from build123d import *

# Parameters (mm, degrees)
SKETCH_1_W               = 250
SKETCH_1_H               = 250
EXTRUDE_1_DEPTH          = 3
HOLE_WIZARD_1_D          = 3.3
PATTERN_CIRCULAR_1_COUNT = 6
SKETCH_5_R               = 22.5
CUT_EXTRUDE_1_DEPTH      = 10


with BuildPart() as part:
    # 草图1 → 凸台-拉伸1 (new body)
    with BuildSketch(Plane(origin=(0, 0, 0), x_dir=(1, 0, 0), z_dir=(0, 1, 0))):
        Rectangle(SKETCH_1_W, SKETCH_1_H)
    extrude(amount=EXTRUDE_1_DEPTH)

    # 孔1 (through all)
    with Locations(Plane(origin=(0, 3, 0), x_dir=(1, 0, 0), z_dir=(0, 1, 0))):
        with Locations((0, -48)):
            hole_wizard_1 = Hole(HOLE_WIZARD_1_D / 2)

    # 阵列(圆周)1: 孔1 ×6 about axis
    pattern_circular_1_axis = Axis((0, 0, 76.5), (0, 1, 0))
    for i in range(1, PATTERN_CIRCULAR_1_COUNT):
        add(hole_wizard_1.rotate(pattern_circular_1_axis, i * 360 / PATTERN_CIRCULAR_1_COUNT), mode=Mode.SUBTRACT)

    # 草图5 → 切除-拉伸1 (cut)
    with BuildSketch(Plane(origin=(0, 3, 0), x_dir=(1, 0, 0), z_dir=(0, 1, 0))):
        with Locations(Location((0, -76.5, 0), (0, 0, 270))):
            Circle(SKETCH_5_R)
    extrude(amount=-CUT_EXTRUDE_1_DEPTH, mode=Mode.SUBTRACT)


solid = part.part
Check sheet for the modelled part. Datum: model origin and axes. Units: mm. Give positions to 0.01 mm unless a question says otherwise; leave off trailing zeros. Loops run counter-clockwise (first coordinate to the right, second up) from the corner with the lowest first, then second, coordinate; pieces in that order, holes last. Notation, with made-up numbers: M 33.25,39.5 L 66.25,39.5 A19 ccw 66.25,74.5 Z; hole C 34.25,-6.5 d7. An arc over 180 degrees is marked long. Use a Markdown table: item, result. Add a question column.
Q1. Scan lines: line 1 along X through (y, z) = (1.2, 105); line 2 along Z through (x, y) = (20.5, 1.55); line 3 along Z through (x, y) = (-1.5, 1.65). Record each from-to range of solid material in increasing order. Write a range as [from, to].
Q2. Sectioned sample at B-B, the plane y = 1.35. Record the cut outline in (x, z).
Q3. Mould release check, pull along Z, two halves, no side actions. Record for faces 1 (the cylindrical face through (0.99, 1.52, 54.02)), 2 (the flat face through (-2, 3, -2)): pulls with the +Z half, pulls with the -Z half, needs draft (parallel to the pull), parting line crosses it, or undercut.
Q4. Sectioned sample at A-A, the plane z = 76.5. Record the cut outline in (x, y), then the cut area to 3 significant figures.
Verdict:
| question | item | result |
|---|---|---|
| 1 | line 1 | [-125, -1.65], [1.65, 125] |
| 1 | line 2 | [-125, 67.23], [85.77, 125] |
| 1 | line 3 | [-125, 47.31], [48.69, 54.05], [98.95, 104.31], [105.69, 125] |
| 2 | outline | M -125,-125 L 125,-125 L 125,125 L -125,125 Z; hole C -24.68,62.25 d3.3; hole C -24.68,90.75 d3.3; hole C 0,76.5 d45; hole C 0,48 d3.3; hole C 0,105 d3.3; hole C 24.68,62.25 d3.3; hole C 24.68,90.75 d3.3 |
| 3 | face 1 | undercut |
| 3 | face 2 | needs draft |
| 4 | outline | M -125,0 L -22.5,0 L -22.5,3 L -125,3 Z; M 22.5,0 L 125,0 L 125,3 L 22.5,3 Z |
| 4 | area | 615 mm^2 |
